Autodesk Inventor part; units mm, degrees
ref_plane "YZ Plane" through (0, 0, 0) normal (1, 0, 0) x (0, 1, 0)
ref_plane "XZ Plane" through (0, 0, 0) normal (0, 1, 0) x (-1, 0, 0)
ref_plane "XY Plane" through (0, 0, 0) normal (0, 0, 1) x (1, 0, 0)
sketch "Sketch1" plane through (0, 0, 0) normal (0, 0, 1) x (1, 0, 0)
  line L0 (0, 0) -> (0, 1910) construction
  line L1 (424.5155, 1910) -> (-415.4845, 1910)
  line L2 (-415.4845, 1910) -> (-1180, 1150)
  line L3 (-1180, 0) -> (-1180, 1150)
  line L4 (960, 0) -> (960, 1342.8524)
  line L5 (424.5155, 1910) -> (960, 1342.8524)
  circle A0 centre (0, 950) radius 195 construction
  line L6 (960, 0) -> (-1180, 0)
  circle A1 centre (-960, 220) radius 200.5
  circle A2 centre (-588, 255) radius 38
  circle A3 centre (374.6358, 1277) radius 50
  circle A4 centre (0, 950) radius 155
  point P0 (0, 955)
  dimension "d1" = 840
  dimension "d3" = 1150
  dimension "d11" = 390
  dimension "d12" = 1180
  dimension "d13" = 950
  dimension "d14" = 76
  dimension "d15" = 1910
  dimension "d16" = 255
  dimension "d17" = 220
  dimension "d18" = 401
  dimension "d19" = 220
  dimension "d21" = 1277
  dimension "d22" = 1554.6358
  dimension "d23" = 100
  dimension "d33" = 2140
  dimension "d34" = 494
  dimension "d45" = 310
  dimension "d49" = 372
  dimension "d51" = 780
  dimension "d52" = 1078
extrude "Extrusion1" add sketch "Sketch1" along normal blind 10
sketch "Sketch3" plane through (0, 0, 10) normal (0, 0, 1) x (1, 0, 0)
  line L0 (-400, 950) -> (400, 950) construction
  circle A0 centre (0, 950) radius 155
  circle A1 centre (155, 950) radius 2.5
  circle A2 centre (-155, 950) radius 2.5
  line L1 (132.7592, 870) -> (-132.7592, 870) construction
  circle A3 centre (132.7592, 870) radius 2.5
  circle A4 centre (-132.7592, 870) radius 2.5
  point P0 (0, 0)
  point P1 (-154.9798, 947.5001)
  point P2 (-154.9798, 952.4999)
  point P3 (154.9798, 947.5001)
  point P4 (154.9798, 952.4999)
  point P5 (134.0322, 872.1516)
  point P6 (131.4516, 867.8692)
  dimension "d47" = 5
  dimension "d48" = 80
extrude "Extrusion3" cut sketch "Sketch3" against normal through all contours A0 A1 | A0 A2 | A3 A0 | A4 A0 | A0 A4 picked at (155.7492, 949.3589) picked at (-155.8257, 950.101) picked at (133.5004, 869.6223)
sketch "Sketch4" plane through (0, 0, 10) normal (0, 0, 1) x (1, 0, 0)
  arc A0 (154.9798, 947.5001) -> (154.9798, 952.4999) centre (155, 950) ccw
  arc A1 (134.0322, 872.1516) -> (154.9798, 947.5001) centre (0, 950) ccw
  arc A2 (131.4516, 867.8692) -> (134.0322, 872.1516) centre (132.7592, 870) ccw
  arc A3 (-131.4516, 867.8692) -> (131.4516, 867.8692) centre (0, 950) ccw
  arc A4 (-134.0322, 872.1516) -> (-131.4516, 867.8692) centre (-132.7592, 870) ccw
  arc A5 (-154.9798, 947.5001) -> (-134.0322, 872.1516) centre (0, 950) ccw
  arc A6 (-154.9798, 952.4999) -> (-154.9798, 947.5001) centre (-155, 950) ccw
  arc A7 (154.9798, 952.4999) -> (-154.9798, 952.4999) centre (0, 950) ccw
  line L0 (960, 1342.8524) -> (424.5155, 1910)
  line L1 (424.5155, 1910) -> (-415.4845, 1910)
  line L2 (-415.4845, 1910) -> (-1180, 1150)
  line L3 (-1180, 1150) -> (-1180, 0)
  line L4 (-1180, 0) -> (960, 0)
  line L5 (960, 0) -> (960, 1342.8524)
  circle A8 centre (374.6358, 1277) radius 50
  circle A9 centre (-588, 255) radius 38
  circle A10 centre (-960, 220) radius 200.5
  line L6 (-380, 0) -> (-380, 1910)
  point P0 (0, 0)
  dimension "d53" = 1340
extrude "Extrusion4" cut sketch "Sketch4" against normal through all contours L5 L4 L6 L1 L0
equation "\"d17\" = d19"
properties part number "ДМФ 014 Стенка Нос ЛЕВ"
Can you work these out from the model? Positions are in its coordinate system, mm. Give positions to 0.01 mm unless a question says otherwise; leave off trailing zeros. Order: outer loops, then holes, each group sorted by start corner. A loop starts at its lowest first (then second) coordinate and runs counter-clockwise, first axis right, second up. Notation, with made-up numbers: M 69,-31.5 L 105,-31.5 A32 cw 105,6.5 Z; hole C 22.25,-38 d2. An arc over 180 degrees is marked long. One line per question, with ' | ' between items.
Item 1: Suppose I cut it at B-B, the plane y = 255. Write out the boundary of the cut face in (x, z), then the cut area to 3 significant figures.
Answer block:
outline: M -1180,0 L -1157.42,0 L -1157.42,10 L -1180,10 Z; M -762.58,0 L -626,0 L -626,10 L -762.58,10 Z; M -550,0 L -380,0 L -380,10 L -550,10 Z | area: 3,290 mm2
Item 2: I'm going to push flat-ended pins straight in: pin 1 Ø4 at (x, z) = (-987, 5) entering from +Y; pin 2 Ø12 at (x, y) = (-466, 1133) entering from -Z; pin 3 Ø2 at (y, z) = (1246.5, 3) entering from -X. Where does each tip first touch, or does it pass through?
Answer block:
pin 1: stops at y = 1343.85 | pin 2: stops at z = 0 | pin 3: stops at x = -1083.93
Item 3: Suppose I cut it at C-C, the plane x = -926.5. Write out the boundary of the cut face in (y, z), then the cut area to 3 significant figures.
Answer block:
outline: M 0,0 L 22.32,0 L 22.32,10 L 0,10 Z; M 417.68,0 L 1402,0 L 1402,10 L 417.68,10 Z | area: 10,100 mm2
Item 4: Suppose I cut it at A-A, the plane z = 3. Write out the boundary of the cut face in (x, y), then the cut area to 3 significant figures.
Answer block:
outline: M -1180,0 L -380,0 L -380,1910 L -415.48,1910 L -1180,1150 Z; hole C -960,220 d401; hole C -588,255 d76 | area: 1,110,000 mm2
Item 5: Please list where these lines run through material, in increasing order: L1, parallel to Y at x = -1107.5, z = 2.75; L2, parallel to Y at x = -588, z = 2; L3, parallel to X at y = 90, z = 1.25.
Answer block:
L1: y = 0 to 84.19, 355.81 to 1222.07 | L2: y = 0 to 217, 293 to 1738.5 | L3: x = -1180 to -1112.64, -807.36 to -380
Item 6: Suppose I cut it at D-D, the plane x = -588. Write out the boundary of the cut face in (y, z), then the cut area to 3 significant figures.
Answer block:
outline: M 0,0 L 217,0 L 217,10 L 0,10 Z; M 293,0 L 1738.5,0 L 1738.5,10 L 293,10 Z | area: 16,600 mm2
Item 7: We'd pull the mould along Y, two halves only. Please class faces 1 (the face through (-1160.306, 211.184, 4.93)), 2 (the face through (-792.39, 1535.32, 4.93)), 3 (the face through (-697, 756, 0)): released by +Y, released by -Y, zero draft, split by the parting line, or undercut.
Answer block:
face 1: undercut | face 2: released by +Y | face 3: zero draft
